from build123d import *

# Parameters (mm, degrees)
F2_R     = 12.5
F3_DEPTH = 40.001


with BuildPart() as f1:
    # F0 (on Front) → F1 (revolve)
    with BuildSketch(Plane.XZ):
        Polygon((-19.310038, 0), (0, 0), (0, 4.444444), (4.014336, 7.885304), (4.014336, 25.089604), (13.189962, 25.089604), (13.189962, 37.849461), (11.612903, 40), (-19.310038, 40), align=None)
    revolve(axis=Axis((-19.310038, 0, 20), (0, 0, -1)))

    # F2 (on face) → F3 (cut, through all)
    with BuildSketch(Plane.XY.offset(40)):
        with Locations((-19.310038, 0)):
            Circle(F2_R)
    extrude(amount=-F3_DEPTH, mode=Mode.SUBTRACT)


solid = f1.part
Can you work these out from the model? Positions are in its coordinate system, mm. A direction names the side the tool comes from. Coordinates: 2 decimals unless noted, no trailing zeros. Write each loop counter-clockwise with the first axis right and the second up, starting at its lowest first coordinate (ties: lowest second). Pieces come first, ordered by that corner, then holes. Notation, with made-up numbers: (-25.5, -9) -> (8.5, -9) arc R13 cw to (8.5, -2) -> close; hole circle Ø6 at (-25.5, 52). An arc over 180 degrees is marked (long way). Answer as CSV lines item,"result".
1) On a 3-axis mill with a long thin cutter (end or side, diameter ignored), from which of +Z, -Z, +X, -X, +Y, -Y can I reach the whole of each face in a straight line? I mean faces 1 (the flat face through (-6, 0, 40)), 2 (the cylindrical face through (2.236, 8.933, 16.608)). Say none if no direction works.
Check result:
face 1,"+Z, +X, -X, +Y, -Y"
face 2,"-Z"
2) If we section it at B-B on z = 28: Please give me the cut outline in (x, y).
Check result:
outline,"circle Ø65 at (-19.31, 0); hole circle Ø25 at (-19.31, 0)"
3) Will these pins go through, and if not, where does the flat tip stop? P1, Ø3, axis at x = -38, z = 10, coming from the -Y side; P2, Ø5, axis at y = -19.5, z = 34.5, coming from the +X side; P3, Ø1, axis at y = -13.5, z = 26, coming from the +X side.
Check result:
P1,"y = -15.76"
P2,"x = 8.39"
P3,"x = 10.48"
4) If we mould it in two halves opening along Y, with no side actions, what happens to faces 3 (the cylindrical face through (-7.4, 3.8, 20.3)), 4 (the flat face through (-19, 13, 0)), 5 (the cylindrical face through (-0.89, -5.8, 2.25))? For each: +Y half, -Y half, draft (parallel to the pull), parting line (faces both ways), or undercut.
Check result:
face 3,"undercut"
face 4,"draft"
face 5,"parting line"
5) If we section it at A-A on y = 0: Please give me the cut outline in (x, z), then the cut area to 3 significant figures.
Check result:
outline,"(-51.81, 25.09) -> (-42.63, 25.09) -> (-42.63, 7.89) -> (-38.62, 4.44) -> (-38.62, 0) -> (-31.81, 0) -> (-31.81, 40) -> (-50.23, 40) -> (-51.81, 37.85) -> close; (-6.81, 0) -> (0, 0) -> (0, 4.44) -> (4.01, 7.89) -> (4.01, 25.09) -> (13.19, 25.09) -> (13.19, 37.85) -> (11.61, 40) -> (-6.81, 40) -> close"
area,"1,090 mm²"
6) If I drill on line 1 (Y direction, x = -19.5, z = 32.5); line 2 (Y direction, x = -39, z = 17.5); line 3 (Z direction, x = -38, y = 21.5), over which ranges is the centre line in solid material (lowest first)? Write a range as from..to.
Check result:
line 1,"-32.5..-12.5, 12.5..32.5"
line 2,"-12.5..12.5"
line 3,"25.09..40"
